Model file for the job. Use its own axes, mm. A direction names the side the tool comes from. Round coordinates to 2 decimals unless told otherwise and drop trailing zeros. Loops run counter-clockwise (first coordinate to the right, second up) from the corner with the lowest first, then second, coordinate; pieces in that order, holes last. Notation, with made-up numbers: (-31.75, 68) -> (-26.75, 68) arc R31 cw to (-26.75, 106) -> close; hole circle Ø3 at (73, -28). An arc over 180 degrees is marked (long way). Use a Markdown table: item, result. Add a question column.
Autodesk Inventor part; units mm, degrees
ref_plane "YZ Plane" through (0, 0, 0) normal (1, 0, 0) x (0, 1, 0)
ref_plane "XZ Plane" through (0, 0, 0) normal (0, 1, 0) x (-1, 0, 0)
ref_plane "XY Plane" through (0, 0, 0) normal (0, 0, 1) x (1, 0, 0)
sketch "Náčrt1" plane through (0, 0, 0) normal (0, 0, 1) x (1, 0, 0)
  line L0 (-5, 8) -> (-5, 0)
  line L1 (-5, 0) -> (5, 0)
  line L2 (5, 0) -> (5, 8)
  line L3 (5, 8) -> (3.5, 8)
  line L4 (3.5, 8) -> (3.5, 1.5)
  line L5 (3.5, 1.5) -> (-3.5, 1.5)
  line L6 (-3.5, 1.5) -> (-3.5, 8)
  line L7 (-3.5, 8) -> (-5, 8)
  line L8 (-7, 0) -> (7, 0)
  line L9 (0, 9.6) -> (0, -1.6)
  point P0 (0, 0)
  dimension "d0" = 10
  dimension "d1" = 8
  dimension "d2" = 1.5
  dimension "d3" = 1.5
  dimension "d4" = 1.5
extrude "Vysunutí1" add sketch "Náčrt1" along normal mid plane 24
sketch "Náčrt2" plane through (0, 0, 12) normal (0, 0, 1) x (1, 0, 0)
  line L0 (-5, 8) -> (-5, 0)
  line L1 (-5, 0) -> (5, 0)
  line L2 (5, 0) -> (5, 8)
  line L3 (5, 8) -> (3.5, 8)
  line L4 (3.5, 8) -> (3.5, 1.5)
  line L5 (3.5, 1.5) -> (-3.5, 1.5)
  line L6 (-3.5, 1.5) -> (-3.5, 8)
  line L7 (-3.5, 8) -> (-5, 8)
  line L8 (-5, 0) -> (5, 0)
  line L9 (5, 0) -> (5, 1.5)
  line L10 (5, 1.5) -> (-5, 1.5)
  line L11 (-5, 1.5) -> (-5, 0)
  line L12 (3.5, 1.5) -> (-3.5, 1.5)
  point P0 (0, 0)
extrude "Vysunutí2" add sketch "Náčrt2" along normal blind 1 contours L10 L5 L2 L1 L0
sketch "Náčrt3" plane through (0, 0, 13) normal (0, 0, 1) x (1, 0, 0)
  line L0 (-5, 1.5) -> (-5, 0)
  line L1 (-5, 0) -> (5, 0)
  line L2 (5, 0) -> (5, 1.5)
  line L3 (5, 1.5) -> (-5, 1.5)
  line L4 (-5, 1.5) -> (-5, 0)
  line L5 (5, 0) -> (-5, 0)
  line L6 (3.5, 1.5) -> (5, 1.5)
  line L7 (5, 1.5) -> (5, 0)
  line L8 (-5, 1.5) -> (-2.7769, 7.608)
  line L9 (-5, 1.5) -> (1.5, 1.5) construction
  line L10 (-2.7769, 7.608) -> (-1.3673, 7.095)
  line L11 (-1.3673, 7.095) -> (-3.4037, 1.5)
  line L12 (0, 9.6) -> (0, -1.6)
  line L13 (5, 1.5) -> (2.7769, 7.608)
  line L14 (2.7769, 7.608) -> (1.3673, 7.095)
  line L15 (1.3673, 7.095) -> (3.4037, 1.5)
  line L16 (-3.4037, 1.5) -> (3.4037, 1.5)
  line L17 (-3.4037, 1.5) -> (3.4037, 1.5)
  point P0 (0, 0)
  dimension "d9" = 6.5
  dimension "d10" = 70
  dimension "d11" = 1.5
extrude "Vysunutí3" add sketch "Náčrt3" along normal blind 5
fillet "Zaoblení1" radius 0.75 8 edges at (-3.5, 8, 0) (-5, 8, 0) (-2.7769, 7.608, 15.5) (-1.3673, 7.095, 15.5) (1.3673, 7.095, 15.5) (2.7769, 7.608, 15.5) (3.5, 8, 0) (5, 8, 0)
sketch "Náčrt4" plane through (5, 0, 18) normal (1, 0, 0) x (0, 0, -1)
  line L0 (6, 7.25) -> (30, 7.25)
  line L1 (6, 1.5) -> (6, 7.25)
  line L2 (6, 1.5) -> (5, 1.5)
  line L3 (5, 1.5) -> (0, 1.5)
  line L4 (0, 0) -> (0, 1.5)
  line L5 (30, 0) -> (0, 0)
  line L6 (30, 7.25) -> (30, 0)
  point P0 (18, 0)
  point P1 (18, 2.75)
  dimension "d15" = 12
  dimension "d16" = 2.75
hole "Díra1" at (5, 2.75, 0) direction (-1, 0, 0) diameter 2.5 end through all
sketch "Náčrt5" plane through (-3.5, 1.5, -12) normal (0, 1, 0) x (1, 0, 0)
  line L0 (7, 0) -> (7, -12)
  line L1 (0, 0) -> (7, 0)
  line L2 (0, 0) -> (0, -12)
  line L3 (0, -12) -> (0, -24)
  line L4 (-1.5, -24) -> (0, -24)
  line L5 (-1.5, -24) -> (-1.5, -25)
  line L6 (0.0963, -25) -> (-1.5, -25)
  line L7 (0.0963, -25) -> (0.0963, -30)
  line L8 (6.9037, -30) -> (0.0963, -30)
  line L9 (6.9037, -25) -> (6.9037, -30)
  line L10 (8.5, -25) -> (6.9037, -25)
  line L11 (8.5, -24) -> (8.5, -25)
  line L12 (7, -24) -> (8.5, -24)
  line L13 (7, -12) -> (7, -24)
  line L14 (-1.5, 0) -> (-1.5, -24)
  point P0 (3.5, -12)
  point P1 (3.5, -6)
  point P2 (3.5, -18)
  dimension "d24" = 5
  dimension "d25" = 6
  dimension "d26" = 12
hole "Díra2" at (0, 1.5, -6) at (0, 1.5, 6) direction (0, -1, 0) diameter 3.2 end through all
properties part number "y_holder" material "Hliník 6061"
1) Tool access for faces 4 (the face through (4.03, 4.16, 15.46)), 5 (the face through (3.5, 4.4, -0.2)), 6 (the face through (-4, 5, 12)), 7 (the face through (2.5, 3.98, 15.46)), 8 (the face through (-4.03, 4.16, 15.46)): list every direction of +Z, -Z, +X, -X, +Y, -Y with a clear straight run to the whole face (end or side of a thin tool).
2) Pull direction Y, two halves, no side cores. Call faces 1 (the face through (1.65, 6.97, 15.54)), 2 (the face through (3, 4, 13)), 3 (the face through (2.7, 7.3, 15.5)): +Y half, -Y half, draft (parallel to the pull), parting line (faces both ways), or undercut.
3) Cut at D-D on y = 5.25. Write the cut outline in (x, z).
4) Wall check: probe 1 along Z at (x, y) = (4.2, 2.75); probe 2 along Z at (x, y) = (0, 0.65); probe 3 along X at (y, z) = (2, -3). Give the ranges that are in metal, low to high. Write a range as from..to.
5) Pin check, flat tips, straight feed: pin 1 Ø6 at (x, z) = (-0.5, 12) entering from -Y; pin 2 Ø2 at (y, z) = (2.75, 0) entering from +X. Stop position of each tip, or through.
6) Cut at A-A on x = 0. Write the cut outline in (y, z), and give its area (3 significant figures).
Established:
| question | item | result |
|---|---|---|
| 1 | face 4 | +Z, +X, +Y |
| 1 | face 5 | -Z, +Y |
| 1 | face 6 | +X, -X, +Y |
| 1 | face 7 | +Z, -Z |
| 1 | face 8 | +Z, -X, +Y |
| 2 | face 1 | undercut |
| 2 | face 2 | draft |
| 2 | face 3 | +Y half |
| 3 | outline | (-5, -12) -> (-3.5, -12) -> (-3.5, 12) -> (-5, 12) -> close; (-3.64, 13) -> (-2.04, 13) -> (-2.04, 18) -> (-3.64, 18) -> close; (2.04, 13) -> (3.64, 13) -> (3.64, 18) -> (2.04, 18) -> close; (3.5, -12) -> (5, -12) -> (5, 12) -> (3.5, 12) -> close |
| 4 | probe 1 | z = -12..-1.25, 1.25..12, 13..18 |
| 4 | probe 2 | z = -12..-7.6, -4.4..4.4, 7.6..18 |
| 4 | probe 3 | x = -5..-3.5, 3.5..5 |
| 5 | pin 1 | stops at y = 0 |
| 5 | pin 2 | passes through |
| 6 | outline | (0, -12) -> (1.5, -12) -> (1.5, -7.6) -> (0, -7.6) -> close; (0, -4.4) -> (1.5, -4.4) -> (1.5, 4.4) -> (0, 4.4) -> close; (0, 7.6) -> (1.5, 7.6) -> (1.5, 18) -> (0, 18) -> close |
| 6 | area | 35.4 mm^2 |
